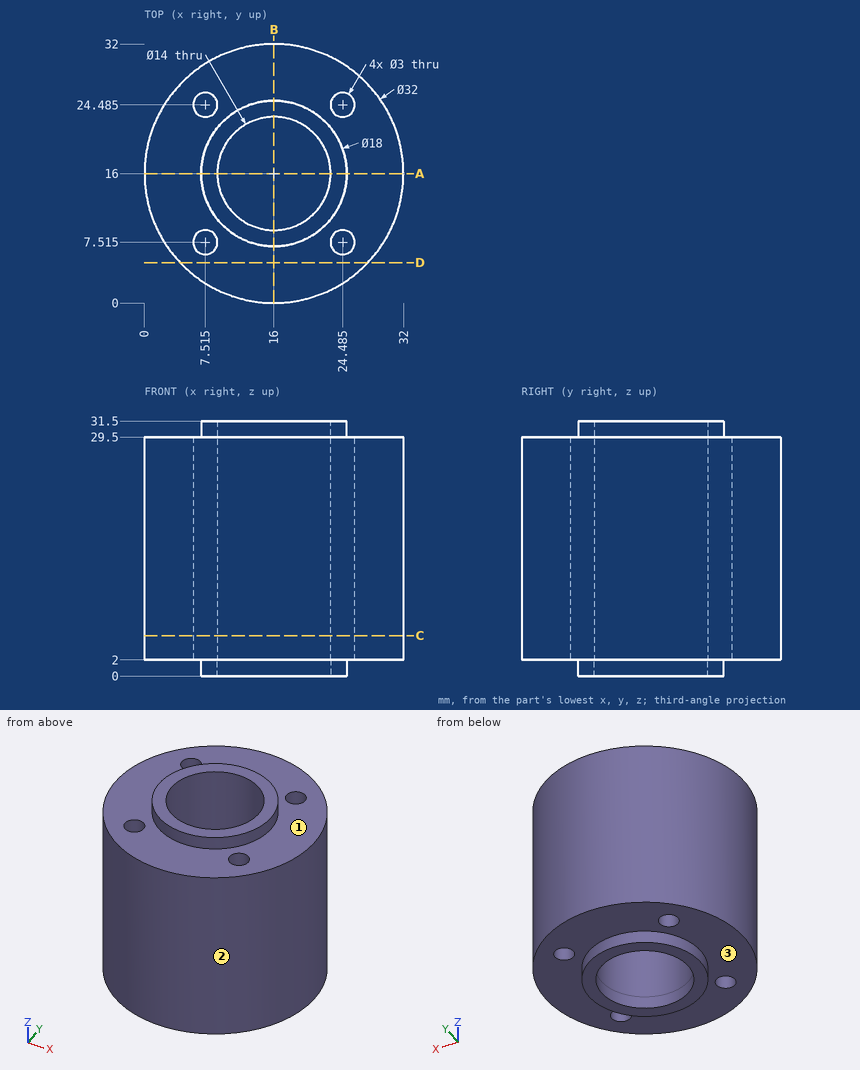
Input: dimensioned drawing with shaded views. Units: mm. Origin: part minimum x, y, z. A direction names the side the tool comes from. Give positions to 0.01 mm unless a question says otherwise; leave off trailing zeros. Write each loop counter-clockwise with the first axis right and the second up, starting at its lowest first coordinate (ties: lowest second). Pieces come first, ordered by that corner, then holes.
Q1. Set-up query: the marked faces 1, 2 and 3. Return all of +Z, -Z, +X, -X, +Y, -Y with unobstructed straight access to the full face (end or side cutting, diameter ignored); none if empty.
Q2. Material intervals for probe 1 along X at (y, z) = (25.5, 26) (1 decimal); probe 2 along Y at (x, z) = (16, 14), sorted ascending.
Q3. First-contact query: P1, Ø2, axis at y = 23, z = 16.5, coming from the +X side; P2, Ø2, axis at y = 10.5, z = 12.5, coming from the +X side; P3, Ø1.5, axis at y = 17, z = 4.5, coming from the +X side. Flat tips, straight axial feed; report the tip coordinate or a pass-through.
Q4. Section C-C, the plane z = 5. Output: boundary loops of the cut face in (x, y) (1 decimal).
Q5. Section D-D, the plane y = 5. Output: boundary loops of the cut face in (x, z), plus the area to 3 significant figures.
Q6. Section A-A, the plane y = 16. Output: boundary loops of the cut face in (x, z).
Filled in:
1. face 1: +Z
1. face 2: +Z, -Z
1. face 3: -Z
2. probe 1: x = 3.1 to 6.4, 8.6 to 23.4, 25.6 to 28.9
2. probe 2: y = 0 to 9, 23 to 32
3. P1: stops at x = 30.83
3. P2: stops at x = 31.35
3. P3: stops at x = 32
4. outline: circle Ø32 at (16, 16); hole circle Ø3 at (7.5, 7.5); hole circle Ø3 at (7.5, 24.5); hole circle Ø14 at (16, 16); hole circle Ø3 at (24.5, 7.5); hole circle Ø3 at (24.5, 24.5)
5. outline: (4.38, 2) - (27.62, 2) - (27.62, 29.5) - (4.38, 29.5) - close
5. area: 639 mm2
6. outline: (0, 2) - (7, 2) - (7, 0) - (9, 0) - (9, 31.5) - (7, 31.5) - (7, 29.5) - (0, 29.5) - close; (23, 0) - (25, 0) - (25, 2) - (32, 2) - (32, 29.5) - (25, 29.5) - (25, 31.5) - (23, 31.5) - close
